The drawing under review shows one solid part. Ordinate dimensions are in mm from its lowest x, y, z. Coordinates: 2 decimals unless noted, no trailing zeros. Order: outer loops, then holes, each group sorted by start corner. A loop starts at its lowest first (then second) coordinate and runs counter-clockwise, first axis right, second up. Notation, with made-up numbers: (48.25, 6) - (78.25, 6) arc R22 ccw to (78.25, 29) - close; hole circle Ø1 at (-10.75, 88.25). An arc over 180 degrees is marked (long way). Write each question's results on one line, items separated by ' | '. Start each with the question number.
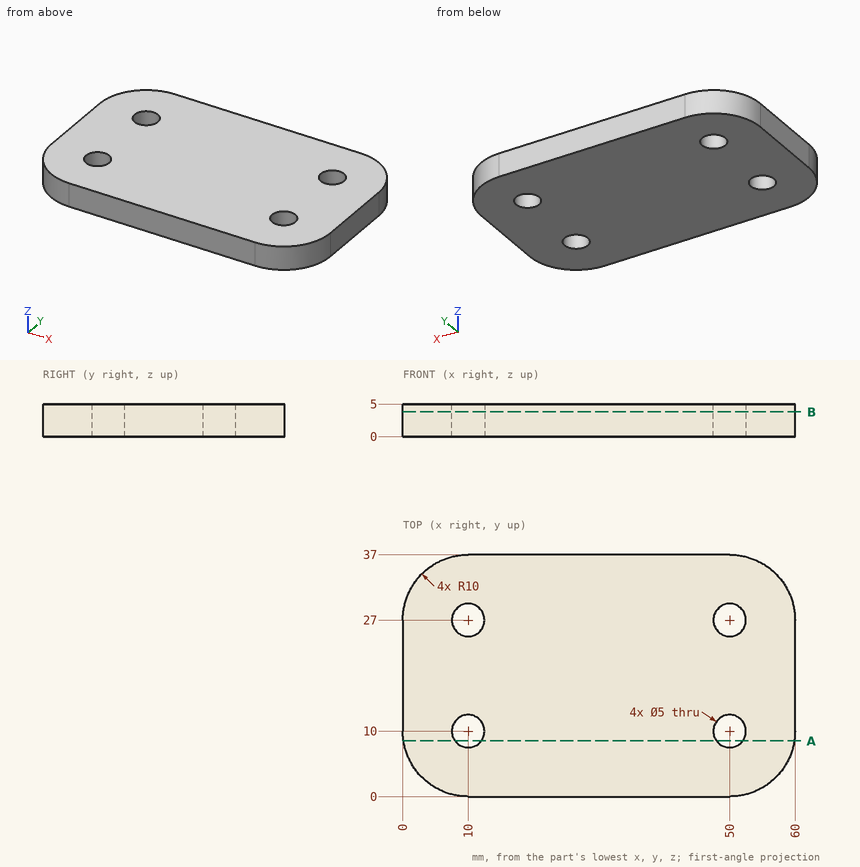
(1) Clearance check with a flat-ended pin moving along its axis: pin 1 (4 mm diameter, centred on x = 10, y = 10, fed in from +Z). State where the tip first meets the part, or that it passes through.
(2) To check wall thickness, follow line 1 along Y through (x, z) = (50, 2.9); line 2 along X through (y, z) = (25, 4.7); line 3 along Y through (x, z) = (49.5, 3.25). State the ranges of each line that lie inside material, in increasing order. Write a range as [from, to].
(3) Take a section at B-B (z = 3.8). State the section outline as (x, y) points, plus the area to 3 significant figures.
(4) Take a section at A-A (y = 8.5). State the section outline as (x, z) points, plus the area to 3 significant figures.
Worked out:
1) pin 1: through
2) line 1: [0, 7.5], [12.5, 24.5], [29.5, 37] | line 2: [0, 8.5], [11.5, 48.5], [51.5, 60] | line 3: [0, 7.55], [12.45, 24.55], [29.45, 37]
3) outline: (0, 10) arc R10 ccw to (10, 0) - (50, 0) arc R10 ccw to (60, 10) - (60, 27) arc R10 ccw to (50, 37) - (10, 37) arc R10 ccw to (0, 27) - close; hole circle Ø5 at (10, 10); hole circle Ø5 at (10, 27); hole circle Ø5 at (50, 10); hole circle Ø5 at (50, 27) | area: 2,060 mm^2
4) outline: (0.11, 0) - (8, 0) - (8, 5) - (0.11, 5) - close; (12, 0) - (48, 0) - (48, 5) - (12, 5) - close; (52, 0) - (59.89, 0) - (59.89, 5) - (52, 5) - close | area: 259 mm^2
